Autodesk Fusion 360 part; units mm, degrees
sketch "Sketch1" plane through (0, 0, 0) normal (0, 0, 1) x (1, 0, 0)
  line L0 (0, 0) -> (106, 0)
  line L1 (106, 0) -> (106, 106)
  line L2 (106, 106) -> (0, 106)
  line L3 (0, 106) -> (0, 0)
  line L4 (2.75, 2.75) -> (103.25, 2.75)
  line L5 (103.25, 2.75) -> (103.25, 103.25)
  line L6 (103.25, 103.25) -> (2.75, 103.25)
  line L7 (2.75, 103.25) -> (2.75, 2.75)
  circle A0 centre (7, 23) radius 4
  circle A1 centre (7, 83) radius 4
  circle A2 centre (99, 23) radius 4
  circle A3 centre (99, 83) radius 4
  line L8 (2.75, 103.25) -> (103.25, 103.25)
  line L9 (103.25, 103.25) -> (103.25, 95.25)
  line L10 (103.25, 95.25) -> (2.75, 95.25)
  line L11 (2.75, 95.25) -> (2.75, 103.25)
  line L12 (2.75, 2.75) -> (103.25, 2.75)
  line L13 (103.25, 2.75) -> (103.25, 10.75)
  line L14 (103.25, 10.75) -> (2.75, 10.75)
  line L15 (2.75, 10.75) -> (2.75, 2.75)
  line L16 (2.75, 95.25) -> (5.75, 95.25)
  line L17 (5.75, 95.25) -> (5.75, 10.75)
  line L18 (5.75, 10.75) -> (2.75, 10.75)
  line L19 (2.75, 10.75) -> (2.75, 95.25)
  line L20 (103.25, 95.25) -> (98.25, 95.25)
  line L21 (98.25, 95.25) -> (98.25, 10.75)
  line L22 (98.25, 10.75) -> (103.25, 10.75)
  line L23 (103.25, 10.75) -> (103.25, 95.25)
  circle A4 centre (7, 83) radius 1.55
  circle A5 centre (99, 83) radius 1.55
  circle A6 centre (7, 23) radius 1.55
  circle A7 centre (99, 23) radius 1.55
  line L24 (103.25, 56) -> (106, 56)
  line L25 (106, 56) -> (106, 44)
  line L26 (106, 44) -> (103.25, 44)
  line L27 (103.25, 44) -> (103.25, 56)
  dimension "d1" = 106
  dimension "d2" = 106
  dimension "d3" = 100.5
  dimension "d4" = 100.5
  dimension "d5" = 2.75
  dimension "d6" = 2.75
  dimension "d7" = 8
  dimension "d8" = 8
  dimension "d9" = 8
  dimension "d10" = 8
  dimension "d12" = 7
  dimension "d13" = 7
  dimension "d16" = 7
  dimension "d17" = 7
  dimension "d18" = 8
  dimension "d19" = 8
  dimension "d20" = 5
  dimension "d21" = 3
  dimension "d22" = 3.1
  dimension "d23" = 3.1
  dimension "d24" = 3.1
  dimension "d25" = 3.1
  dimension "d48" = 23
  dimension "d49" = 23
  dimension "d50" = 23
  dimension "d51" = 23
  dimension "d52" = 12
  dimension "d55" = 41.25
extrude "Extrude1" add sketch "Sketch1" against normal blind 2 contours L0 L1 L2 L3 L4 L5 L6 L7 L8 L9 L11 L12 L13 L15 L19 L23 L24 L26 | L1 L5 L23 L24 L25 L26 L27 | L5 A2 A3 L10 L14 L20 L21 L22 L23 L27 | L4 L5 L7 L12 L13 L14 L15 L18 L22 | L5 L6 L7 L8 L9 L10 L11 L16 L20 | A0 A1 A2 A3 L10 L14 L17 L21 | L7 A0 A1 L10 L14 L16 L17 L18 L19 | A2 L21 A7 | A2 L21 A7 | A3 L21 A5 | A3 L21 A5 | A0 L17 A6 | A0 L17 A6 | A1 L17 A4 | A1 L17 A4
extrude "Extrude2" add sketch "Sketch1" along normal blind 4.6 contours L0 L1 L2 L3 L4 L5 L6 L7 L8 L9 L11 L12 L13 L15 L19 L23 L24 L26
extrude "Extrude3" add sketch "Sketch1" along normal blind 3 contours L1 L5 L23 L24 L25 L26 L27 | L5 A2 A3 L10 L14 L20 L21 L22 L23 L27 | L4 L5 L7 L12 L13 L14 L15 L18 L22 | L5 L6 L7 L8 L9 L10 L11 L16 L20 | L7 A0 A1 L10 L14 L16 L17 L18 L19 | A2 L21 A7 | A2 L21 A7 | A3 L21 A5 | A3 L21 A5 | A0 L17 A6 | A0 L17 A6 | A1 L17 A4 | A1 L17 A4
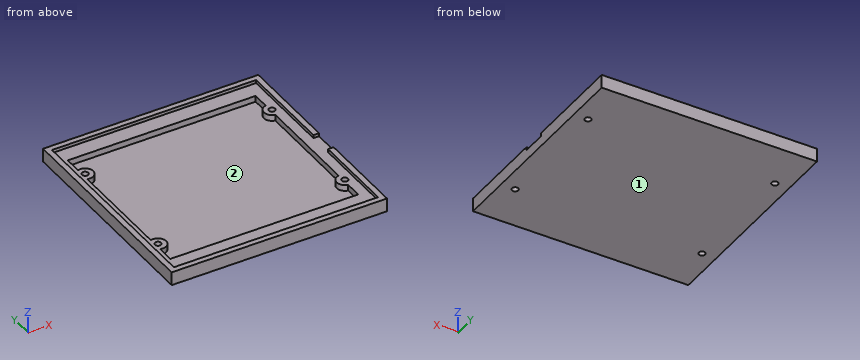
Read the model definition and answer for the solid it produces. Units are mm, in the model's axes. Face numbers are marked on the shaded views. Give positions to 0.01 mm unless a question says otherwise; leave off trailing zeros. Write each loop counter-clockwise with the first axis right and the second up, starting at its lowest first coordinate (ties: lowest second). Pieces come first, ordered by that corner, then holes. Notation, with made-up numbers: (67.5, 67.25) - (97.5, 67.25) arc R15 cw to (97.5, 93.25) - close; hole circle Ø3 at (63, -37). An arc over 180 degrees is marked (long way). Write item = value, one per line. Start each with the question number.
Item 1: Find section C-C (z = 1.75). Give the vertices of the cut face in (x, y), then the cut area to 3 significant figures.
Item 2: The mould has two halves that part along Y. Classify the marked faces 1 and 2: +Y half, -Y half, draft (parallel to the pull), parting line (faces both ways), or undercut.
Item 3: Each of these flat-tipped pins is pushed along its axis until it touches: P1, Ø0.8, axis at x = 104, z = 4, coming from the -Y side; P2, Ø1.5, axis at x = 27.5, y = 32.5, coming from the +Z side; P3, Ø5, axis at x = 99, y = 83, coming from the +Z side. Where does it stop, or does it pass through?
Item 4: Find section D-D (x = 64). Give the vertices of the cut face in (y, z).
Item 5: Find section B-B (x = 7). Give the vertices of the cut face in (y, z).
Item 6: Find the intervals of material crossed by probe 1 along X at (y, z) = (83, -0.55); probe 2 along Y at (x, z) = (7, -0.75); probe 3 along X at (y, z) = (47, 2.5), in increasing order. Write a range as [from, to].
Item 7: Find section A-A (y = 23). Give the vertices of the cut face in (x, z), then the cut area to 3 significant figures.
Response:
q1.outline = (0, 0) - (106, 0) - (106, 106) - (0, 106) - close; hole circle Ø3.1 at (7, 23); hole circle Ø3.1 at (7, 83); hole (5.75, 10.75) - (98.25, 10.75) - (98.25, 19.07) arc R4 cw to (98.25, 26.93) - (98.25, 79.07) arc R4 cw to (98.25, 86.93) - (98.25, 95.25) - (5.75, 95.25) - (5.75, 86.8) arc R4 cw (long way) to (5.75, 79.2) - (5.75, 26.8) arc R4 cw (long way) to (5.75, 19.2) - close; hole circle Ø3.1 at (99, 23); hole circle Ø3.1 at (99, 83)
q1.area = 3,500 mm²
q2.face_1 = draft
q2.face_2 = undercut
q3.P1 = 0
q3.P2 = 0
q3.P3 = 3
q4.outline = (0, -2) - (106, -2) - (106, 4.6) - (103.25, 4.6) - (103.25, 3) - (95.25, 3) - (95.25, 0) - (10.75, 0) - (10.75, 3) - (2.75, 3) - (2.75, 4.6) - (0, 4.6) - close
q5.outline = (0, -2) - (21.45, -2) - (21.45, 3) - (19, 3) - (19, 0) - (10.75, 0) - (10.75, 3) - (2.75, 3) - (2.75, 4.6) - (0, 4.6) - close; (24.55, -2) - (81.45, -2) - (81.45, 3) - (79, 3) - (79, 0) - (27, 0) - (27, 3) - (24.55, 3) - close; (84.55, -2) - (106, -2) - (106, 4.6) - (103.25, 4.6) - (103.25, 3) - (95.25, 3) - (95.25, 0) - (87, 0) - (87, 3) - (84.55, 3) - close
q6.probe_1 = [0, 5.45], [8.55, 97.45], [100.55, 106]
q6.probe_2 = [0, 21.45], [24.55, 81.45], [84.55, 106]
q6.probe_3 = [0, 5.75], [98.25, 106]
q7.outline = (0, -2) - (5.45, -2) - (5.45, 3) - (2.75, 3) - (2.75, 4.6) - (0, 4.6) - close; (8.55, -2) - (97.45, -2) - (97.45, 3) - (95, 3) - (95, 0) - (11, 0) - (11, 3) - (8.55, 3) - close; (100.55, -2) - (106, -2) - (106, 4.6) - (103.25, 4.6) - (103.25, 3) - (100.55, 3) - close
q7.area = 256 mm²
